Geometry check sheet. Reference: the model listing, model coordinates, mm. A direction names the side the tool comes from. Coordinates: 2 decimals unless noted, no trailing zeros. Order: outer loops, then holes, each group sorted by start corner. A loop starts at its lowest first (then second) coordinate and runs counter-clockwise, first axis right, second up. Notation, with made-up numbers: M -23.5,26.5 L 13.5,26.5 A32 ccw 13.5,58.5 Z; hole C -32,-27 d6. An arc over 180 degrees is marked long. One line per item, written item: value. Start each with the question number.
1) Draft check along Z on faces 1 (the flat face through (2.8, 0, 5.2)), 2 (the cylindrical face through (0.249, 0.493, -7.546)), 3 (the cylindrical face through (-0.22, 0.493, -5.746)), 4 (the cylindrical face through (2.54, 0.507, 8.377)). Enter one of: pulls with the +Z half, pulls with the -Z half, needs draft (parallel to the pull), parting line crosses it, or undercut.
2) Sectioned sample at A-A, the plane z = 0. Enter the section's corners in (x, y), then the cut area to 3 significant figures.
3) Sectioned sample at D-D, the plane z = -5.5. Enter the section's corners in (x, y).
4) Sectioned sample at C-C, the plane x = 4. Enter the section's corners in (y, z), then the cut area to 3 significant figures.
5) Thickness scan on L1, parallel to Z at x = 3.25, y = 0.4; L2, parallel to Z at x = 2.75, y = 0.85; L3, parallel to X at y = 0.25, z = 0. Record the ranges inside material, lowest first. Write a range as from..to.
6) Sectioned sample at B-B, the plane y = 0.55. Enter the section's corners in (x, z).
7) Access from +Z, -Z, +X, -X, +Y, -Y to the whole of each face (thin tool, end or side, straight path). Record for faces 5 (the flat face through (-1.908, 0.493, 7.121)), 6 (the flat face through (2.8, 1, 5.2)), 7 (the cylindrical face through (-1.79, 0.51, 5.76)).
```python
from build123d import *

# Parameters (mm, degrees)
SKETCH1_R           = 0.85
BOSS_EXTRUDE1_DEPTH = 1
FILLET1_R           = 1


with BuildPart() as part:
    # Sketch1 → Boss-Extrude1 (new body)
    with BuildSketch(Plane(origin=(0, 0, 0), x_dir=(1, 0, 0), z_dir=(0, 1, 0))):
        with BuildLine():
            Line((-2.342312358, -8.741628728), (-1.488209509, -5.554073501))
            ThreePointArc((-1.488209509, -5.554073501), (0, 5.75), (1.488209509, -5.554073501))
            Line((1.488209509, -5.554073501), (2.342312358, -8.741628728))
            Line((2.342312358, -8.741628728), (5.529867585, -7.887525879))
            Line((5.529867585, -7.887525879), (4.94509663, -5.705130964))
            ThreePointArc((4.94509663, -5.705130964), (0, 7.55), (-4.94509663, -5.705130964))
            Line((-4.94509663, -5.705130964), (-5.529867585, -7.887525879))
            Line((-5.529867585, -7.887525879), (-2.342312358, -8.741628728))
        make_face()
        with Locations((-3.509038547, -6.72079969)):
            Circle(SKETCH1_R, mode=Mode.SUBTRACT)
        with Locations((3.509038547, -6.72079969)):
            Circle(SKETCH1_R, mode=Mode.SUBTRACT)
    extrude(amount=BOSS_EXTRUDE1_DEPTH)

    # Fillet1
    fillet1_edges = [part.edges().sort_by_distance(p)[0] for p in [
        (5.529867585, 0.5, 7.887525879),
        (2.342312358, 0.5, 8.741628728),
        (1.488209509, 0.5, 5.554073501),
        (-1.488209509, 0.5, 5.554073501),
        (-2.342312358, 0.5, 8.741628728),
        (-5.529867585, 0.5, 7.887525879),
        (-4.94509663, 0.5, 5.705130964),
        (4.94509663, 0.5, 5.705130964),
    ]]
    fillet(fillet1_edges, radius=FILLET1_R)


solid = part.part
```
Final values:
1. face 1: needs draft
1. face 2: parting line crosses it
1. face 3: undercut
1. face 4: pulls with the +Z half
2. outline: M -7.55,0 L -5.75,0 L -5.75,1 L -7.55,1 Z; M 5.75,0 L 7.55,0 L 7.55,1 L 5.75,1 Z
2. area: 3.60 mm^2
3. outline: M -5.17,0 L -1.68,0 L -1.68,1 L -5.17,1 Z; M 1.68,0 L 5.17,0 L 5.17,1 L 1.68,1 Z
4. outline: M 0,-6.4 L 1,-6.4 L 1,-4.13 L 0,-4.13 Z; M 0,4.13 L 1,4.13 L 1,6.03 L 0,6.03 Z; M 0,7.41 L 1,7.41 L 1,8.3 L 0,8.3 Z
4. area: 5.05 mm^2
5. L1: z = -6.81..-4.74, 4.74..5.91, 7.53..8.5
5. L2: z = -7.03..-5.05, 5.05..6.34, 7.1..8.47
5. L3: x = -7.55..-5.75, 5.75..7.55
6. outline: M -5.36,5.32 A7.55 ccw long 5.36,5.32 A1 cw 5.1,6.28 L 5.27,6.92 A1 ccw 4.56,8.15 L 3.31,8.48 A1 ccw 2.08,7.78 L 1.73,6.45 A1 ccw 2.29,5.27 A5.75 cw long -2.29,5.27 A1 ccw -1.73,6.45 L -2.08,7.78 A1 ccw -3.31,8.48 L -4.56,8.15 A1 ccw -5.27,6.92 L -5.1,6.28 A1 cw Z; hole C -3.51,6.72 d1.7; hole C 3.51,6.72 d1.7
7. face 5: +Z, +Y, -Y
7. face 6: +Z, -Z, +X, -X, +Y
7. face 7: +Y, -Y
